```python
from build123d import *

# Parameters (mm, degrees)
SKETCH_1_R      = 0.75
EXTRUDE_1_DEPTH = 25
SKETCH_3_R      = 0.75
EXTRUDE_2_DEPTH = 6


with BuildPart() as part:
    # 草图1 → 凸台-拉伸1 (new body)
    with BuildSketch(Plane(origin=(0, 0, 0), x_dir=(1, 0, 0), z_dir=(0, 1, 0))):
        with Locations(Location((0, 0, 0), (0, 0, 270))):
            Circle(SKETCH_1_R)
    extrude(amount=EXTRUDE_1_DEPTH)

    # 草图2 → 旋转1 (revolve)
    with BuildSketch(Plane.XY):
        with BuildLine():
            Line((0, 25.75), (0, 24.25))
            ThreePointArc((0, 24.25), (0.75, 25), (0, 25.75))
        make_face()
    revolve(axis=Axis((0, 25.75, 0), (0, -1, 0)))

    # 草图3 → 凸台-拉伸2 (add)
    with BuildSketch(Plane(origin=(0, 0, 0), x_dir=(0, 0, -1), z_dir=(1, 0, 0))):
        with Locations((0, 25)):
            Circle(SKETCH_3_R)
    extrude(amount=EXTRUDE_2_DEPTH)

    # 草图4 → 旋转2 (revolve)
    with BuildSketch(Plane(origin=(6, 0, 0), x_dir=(0, 0, -1), z_dir=(1, 0, 0))):
        with BuildLine():
            Line((0, 25.75), (0, 24.25))
            ThreePointArc((0, 24.25), (0.75, 25), (0, 25.75))
        make_face()
    revolve(axis=Axis((6, 25.75, 0), (0, -1, 0)))


solid = part.part
```
For this review, take the finished solid that the model builds, in its own axes (mm). A direction names the side the tool comes from. Give positions to 0.01 mm unless a question says otherwise; leave off trailing zeros. Order: outer loops, then holes, each group sorted by start corner. A loop starts at its lowest first (then second) coordinate and runs counter-clockwise, first axis right, second up.
1) Wall thickness on line 1 (Y direction, x = 4.25, z = 0.05); line 2 (Y direction, x = -0.5, z = -0.4); line 3 (Z direction, x = 0.5, y = 22.75): over which ranges is each line inside the solid? List them lowest first.
2) Take a section at B-B (y = 17.25). Give the boundary of the cut face in (x, z), then the cut area to 3 significant figures.
3) Take a section at A-A (z = 0). Give the boundary of the cut face in (x, y).
4) For faces 1 (the face through (2.958, 25.632, -0.403)), 2 (the face through (0.225, 12.325, 0.715)), 3 (the face through (0, 0, 0)), list the 3-axis set-ups (+Z, -Z, +X, -X, +Y, -Y) from which the entire face can be reached by the end or side of a thin tool; tool diameter is ignored.
5) Take a section at C-C (x = 4.75). Give the boundary of the cut face in (y, z).
6) Insertion check: pin 1 (3 mm diameter, centred on x = 2, y = 19, fed in from +Z). The pin has a flat end and moves straight along its axis. Give the tip position at first contact, or say it passes through.
Derived:
1. line 1: y = 24.25 to 25.75
1. line 2: y = 0 to 25.39
1. line 3: z = -0.56 to 0.56
2. outline: circle Ø1.5 at (0, 0)
2. area: 1.77 mm2
3. outline: (-0.75, 0) - (0.75, 0) - (0.75, 24.25) - (6, 24.25) arc R0.75 ccw to (6, 25.75) - (0, 25.75) arc R0.75 ccw to (-0.75, 25) - close
4. face 1: +X
4. face 2: -Y
4. face 3: +Z, -Z, +X, -X, -Y
5. outline: circle Ø1.5 at (25, 0)
6. pin 1: stops at z = 0.56
